Design review of the part built by this model. Coordinates are the model's own, in mm. A direction names the side the tool comes from. Give positions to 0.01 mm unless a question says otherwise; leave off trailing zeros. Order: outer loops, then holes, each group sorted by start corner. A loop starts at its lowest first (then second) coordinate and runs counter-clockwise, first axis right, second up. Notation, with made-up numbers: (10.25, 1) -> (33.25, 1) arc R20 ccw to (33.25, 31) -> close; hole circle Ø8 at (74, 18.25). An arc over 180 degrees is marked (long way). Use a Markdown table: item, result. Add a question column.
Autodesk Inventor part; units mm, degrees
ref_plane "YZ Plane" through (0, 0, 0) normal (1, 0, 0) x (0, 1, 0)
ref_plane "XZ Plane" through (0, 0, 0) normal (0, 1, 0) x (-1, 0, 0)
ref_plane "XY Plane" through (0, 0, 0) normal (0, 0, 1) x (1, 0, 0)
sketch "Náčrt1" plane through (0, 0, 0) normal (0, 0, 1) x (1, 0, 0)
  line L0 (4.5, 0) -> (4.5, -4.5)
  line L1 (4.5, -4.5) -> (-4.5, -4.5)
  line L2 (-4.5, -4.5) -> (-4.5, 4.5)
  line L3 (-4.5, 4.5) -> (4.5, 4.5)
  line L4 (4.5, 4.5) -> (4.5, -4.5)
  circle A0 centre (0, 0) radius 3
  circle A1 centre (0, 0) radius 1.5
  dimension "d1" = 4.5
  dimension "d2" = 9
  dimension "d3" = 9
  dimension "d4" = 9
  dimension "d5" = 6
  dimension "d6" = 3
extrude "Vysunutí1" add sketch "Náčrt1" along normal blind 9 contours L0 L1 L2 L3 L4 | A0 | A1
sketch "Náčrt2" plane through (0, 0, 9) normal (0, 0, 1) x (1, 0, 0)
  circle A0 centre (0, 0) radius 3
  circle A1 centre (0, 0) radius 1.5
  dimension "d9" = 6
  dimension "d10" = 3
extrude "Vysunutí2" add sketch "Náčrt2" along normal blind 3
sketch "Náčrt3" plane through (0, 0, 0) normal (0, 0, -1) x (-1, 0, 0)
  circle A0 centre (0, 0) radius 3
  circle A1 centre (0, 0) radius 1.5
  dimension "d13" = 6
  dimension "d14" = 3
extrude "Vysunutí3" add sketch "Náčrt3" along normal blind 3
sketch "Náčrt4" plane through (-4.5, -4.5, 0) normal (-1, 0, 0) x (0, 0, 1)
  line L0 (0, 9) -> (0, 0)
  line L1 (0, 0) -> (9, 0)
  line L2 (1.5, 0) -> (1.5, 1.5)
  line L3 (1.5, 1.5) -> (1.5, 7.5)
  line L4 (1.5, 7.5) -> (7.5, 7.5)
  line L5 (7.5, 7.5) -> (7.5, 1.5)
  line L6 (7.5, 1.5) -> (1.5, 1.5)
  point P0 (0, 4.5)
  dimension "d18" = 1.5
  dimension "d19" = 6
  dimension "d20" = 6
  dimension "d21" = 6
extrude "Vysunutí4" cut sketch "Náčrt4" against normal blind 9
properties part number "Osa_rameno _1"
1) For L1, parallel to Y at x = 0, z = -2.1; L2, parallel to Y at x = 0, z = 4; L3, parallel to Z at x = 1.25, y = 1.5, list the stretches that pass through material, from the lowest coordinate up. Write a range as [from, to].
2) Machinability: for faces 1 (the flat face through (-3, 1, 9)), 2 (the flat face through (0, 0, 0)), 3 (the flat face through (0, 3, 4)), which of the approach directions +Z, -Z, +X, -X, +Y, -Y give a long, thin tool a straight path to every point of the face, cutting with its end or side? Answer none if there is none.
3) Add section D-D (y = -2). Give the boundary of the cut face in (x, z).
4) Add section A-A (z = 4.5). Give the boundary of the cut face in (x, y), then the cut area to 3 significant figures.
5) Add section C-C (x = 0). Give the boundary of the cut face in (y, z), then the cut area to 3 significant figures.
6) Add section B-B (y = 0). Give the boundary of the cut face in (x, z), then the cut area to 3 significant figures.
7) The part is to be moulded in two halves that separate along X. For faces 4 (the cylindrical face through (3, 0, -1)), 5 (the cylindrical face through (-1.5, -0.07, 10.48)), 6 (the flat face through (0, -4.5, 4)), 7 (the flat face through (0, 0, 9)), say which applies: +X half, -X half, draft (parallel to the pull), parting line (faces both ways), or undercut.
8) Insertion check: pin 1 (3.5 mm diameter, centred on x = 0, y = 0, fed in from +Z). The pin has a flat end and moves straight along its axis. Give the tip position at first contact, or say it passes through.
Worked answers:
| question | item | result |
|---|---|---|
| 1 | L1 | [-3, -1.5], [1.5, 3] |
| 1 | L2 | [-4.5, -3], [3, 4.5] |
| 1 | L3 | [-3, 1.5], [7.5, 12] |
| 2 | face 1 | +Z |
| 2 | face 2 | -Z |
| 2 | face 3 | +X, -X |
| 3 | outline | (-4.5, 0) -> (-2.24, 0) -> (-2.24, -3) -> (2.24, -3) -> (2.24, 0) -> (4.5, 0) -> (4.5, 1.5) -> (-4.5, 1.5) -> close; (-4.5, 7.5) -> (4.5, 7.5) -> (4.5, 9) -> (2.24, 9) -> (2.24, 12) -> (-2.24, 12) -> (-2.24, 9) -> (-4.5, 9) -> close |
| 4 | outline | (-4.5, -4.5) -> (4.5, -4.5) -> (4.5, -3) -> (-4.5, -3) -> close; (-4.5, 3) -> (4.5, 3) -> (4.5, 4.5) -> (-4.5, 4.5) -> close |
| 4 | area | 27.0 mm^2 |
| 5 | outline | (-4.5, 0) -> (-3, 0) -> (-3, -3) -> (-1.5, -3) -> (-1.5, 0) -> (1.5, 0) -> (1.5, -3) -> (3, -3) -> (3, 0) -> (4.5, 0) -> (4.5, 9) -> (3, 9) -> (3, 12) -> (1.5, 12) -> (1.5, 9) -> (-1.5, 9) -> (-1.5, 12) -> (-3, 12) -> (-3, 9) -> (-4.5, 9) -> close; hole (-3, 1.5) -> (3, 1.5) -> (3, 7.5) -> (-3, 7.5) -> close |
| 5 | area | 63.0 mm^2 |
| 6 | outline | (-4.5, 0) -> (-3, 0) -> (-3, -3) -> (-1.5, -3) -> (-1.5, 0) -> (1.5, 0) -> (1.5, -3) -> (3, -3) -> (3, 0) -> (4.5, 0) -> (4.5, 1.5) -> (-4.5, 1.5) -> close; (-4.5, 7.5) -> (4.5, 7.5) -> (4.5, 9) -> (3, 9) -> (3, 12) -> (1.5, 12) -> (1.5, 9) -> (-1.5, 9) -> (-1.5, 12) -> (-3, 12) -> (-3, 9) -> (-4.5, 9) -> close |
| 6 | area | 45.0 mm^2 |
| 7 | face 4 | parting line |
| 7 | face 5 | undercut |
| 7 | face 6 | draft |
| 7 | face 7 | undercut |
| 8 | pin 1 | z = 12 |
